Check sheet for the modelled part. Datum: model origin and axes. Units: mm. A direction names the side the tool comes from. Give positions to 0.01 mm unless a question says otherwise; leave off trailing zeros. Write each loop counter-clockwise with the first axis right and the second up, starting at its lowest first coordinate (ties: lowest second). Pieces come first, ordered by that corner, then holes. Notation, with made-up numbers: M 33.5,-31 L 37.5,-31 A14 cw 37.5,-13 Z; hole C -5.75,-12 d8. An arc over 180 degrees is marked long. Write item = value, one per line. Start each with the question number.
1) Mould release check, pull along X, two halves, no side actions. Record for faces 1 (the flat face through (4.4, 8.255, -0.1)), 2 (the flat face through (1.905, 4, -5)), 3 (the cylindrical face through (-0.07, 0.63, -11.43)): released by +X, released by -X, zero draft, split by the parting line, or undercut.
2) Access from +Z, -Z, +X, -X, +Y, -Y to the whole of each face (thin tool, end or side, straight path). Record for faces 4 (the cylindrical face through (-6.35, 3.93, 0.11)), 5 (the cylindrical face through (6.35, 3.93, -0.11)), 6 (the flat face through (1.905, 4, 5)).
3) Cross-section at A-A, the plane x = 0. Record the cut outline in (y, z), plus the area to 3 significant figures.
4) Scan lines: line 1 along Z through (x, y) = (0, 0.8); line 2 along Y through (x, z) = (-1, 3.5); line 3 along Z through (x, y) = (-3.5, 4). Record each from-to range of solid material in increasing order. Write a range as [from, to].
5) Go/stop test with flat-tipped pins: pin 1 (1.1 mm diameter, centred on y = 5.5, z = -5.5, fed in from -X); pin 2 (1.5 mm diameter, centred on x = 0, z = -6.731, fed in from +Y); pin 3 (0.7 mm diameter, centred on y = 2.5, z = -5.5, fed in from +X); pin 4 (1.6 mm diameter, centred on y = 4, z = 5.5, fed in from -X). Record where each tip stops, or that it passes through.
Autodesk Inventor part; units mm, degrees
ref_plane "Work Plane1" through (0, 8.255, 0) normal (0, 1, 0) x (1, 0, 0)
ref_plane "YZ Plane" through (0, 0, 0) normal (1, 0, 0) x (0, 1, 0)
ref_plane "XZ Plane" through (0, 0, 0) normal (0, 1, 0) x (-1, 0, 0)
sketch "Sketch1" plane through (0, 0, 0) normal (0, 1, 0) x (-1, 0, 0)
  arc A0 (-4.4691, 4.5111) -> (4.4691, 4.5111) centre (0, 0) ccw
  arc A1 (3.1656, 8.0108) -> (-3.1656, 8.0108) centre (0, 8.255) ccw
  circle A2 centre (0, -8.255) radius 3.175
  line L0 (0, 0) -> (3.175, 0)
  arc A3 (3.1656, 8.0108) -> (4.4691, 4.5111) centre (7.5974, 7.6688) ccw
  arc A4 (-4.4691, 4.5111) -> (-3.1656, 8.0108) centre (-7.5974, 7.6688) ccw
  arc A5 (-3.1656, -8.0108) -> (-4.4691, -4.5111) centre (-7.5974, -7.6688) ccw
  arc A6 (4.4691, -4.5111) -> (3.1656, -8.0108) centre (7.5974, -7.6688) ccw
  dimension "d0" = 12.7
  dimension "d2" = 6.35
  dimension "d4" = 6.35
  dimension "d5" = 8.89
  dimension "d6" = 16.51
extrude "Extrusion1" add sketch "Sketch1" along normal blind 1.27
sketch "Sketch2" plane through (0, 1.27, 0) normal (0, 1, 0) x (1, 0, 0)
  line L0 (1.905, -7.3814) -> (-1.905, -7.3814)
  line L1 (-1.905, -7.3814) -> (-1.905, 7.3814)
  line L2 (-1.905, 7.3814) -> (1.905, 7.3814)
  line L3 (1.905, 7.3814) -> (1.905, -7.3814)
  line L4 (1.905, -7.3814) -> (-1.905, 7.3814) construction
  line L5 (-1.905, -7.3814) -> (1.905, 7.3814) construction
  arc A0 (1.905, -4.6407) -> (1.905, 4.6407) centre (0, 0) ccw
  arc A1 (-1.905, 4.6407) -> (-1.905, -4.6407) centre (0, 0) ccw
  arc A2 (1.905, -6.0575) -> (1.905, 6.0575) centre (0, 0) ccw
  arc A3 (-1.905, 6.0575) -> (-1.905, -6.0575) centre (0, 0) ccw
  dimension "d11" = 3.81
  dimension "d34" = 5.0165
  dimension "d35" = 6.35
  dimension "d36" = 5.0165
  dimension "d37" = 6.35
extrude "Extrusion2" add sketch "Sketch2" along normal blind 5.3975 contours L3 A0 A2 | A3 L1 A1
sketch "Sketch3" plane through (0, 6.6675, 0) normal (0, 1, 0) x (1, 0, 0)
  arc A0 (-1.905, 4.6407) -> (-1.905, -4.6407) centre (0, 0) ccw
  line L0 (-1.905, 4.6407) -> (-1.905, 6.0575)
  arc A1 (-1.905, 6.0575) -> (-1.905, -6.0575) centre (0, 0) ccw
  line L1 (-1.905, -6.0575) -> (-1.905, -4.6407)
  line L2 (1.905, -4.6407) -> (1.905, -6.0575)
  arc A2 (1.905, -6.0575) -> (1.905, 6.0575) centre (0, 0) ccw
  line L3 (1.905, 6.0575) -> (1.905, 4.6407)
  arc A3 (1.905, -4.6407) -> (1.905, 4.6407) centre (0, 0) ccw
ref_plane "Work Plane1" through (0, 8.255, 0) normal (0, 1, 0) x (1, 0, 0)
sketch "Sketch4" plane through (0, 8.255, 0) normal (0, 1, 0) x (1, 0, 0)
  arc A0 (0.508, -4.9907) -> (0.508, 4.9907) centre (0, 0) ccw
  arc A1 (0.508, -4.0961) -> (0.508, 4.0961) centre (0, 0) ccw
  line L0 (0.508, -4.9907) -> (0.508, -4.0961)
  line L1 (0.508, 4.0961) -> (0.508, 4.9907)
sketch "Sketch5" plane through (0, 8.255, 0) normal (0, 1, 0) x (1, 0, 0)
  line L0 (-0.508, -4.0961) -> (-0.508, -4.9907)
  arc A0 (-0.508, 4.0961) -> (-0.508, -4.0961) centre (0, 0) ccw
  arc A1 (-0.508, 4.9907) -> (-0.508, -4.9907) centre (0, 0) ccw
  line L1 (-0.508, 4.0961) -> (-0.508, 4.9907)
loft "Loft1" add profiles "Sketch4" section 1 edges at (1.905, 6.6675, 5.3491) (6.35, 6.6675, 0) (1.905, 6.6675, -5.3491) (5.0165, 6.6675, 0)
loft "Loft2" add profiles "Sketch5" section 1 edges at (-5.0165, 6.6675, 0) (-1.905, 6.6675, -5.3491) (-6.35, 6.6675, 0) (-1.905, 6.6675, 5.3491)
sketch "Sketch6" plane through (0, 1.27, 0) normal (0, 1, 0) x (1, 0, 0)
  line L0 (0, 0) -> (-3.0006, 0)
  point P0 (0, -6.731)
  point P1 (0, 6.731)
  dimension "d26" = 13.462
hole "Hole1" at (0, 1.27, 6.731) at (0, 1.27, -6.731) direction (0, -1, 0) diameter 2.4384 end through all
properties part number "CasterEnclosure" material "ABS Plastic"
Reply:
q1.face_1 = zero draft
q1.face_2 = undercut
q1.face_3 = split by the parting line
q2.face_4 = -X, +Y
q2.face_5 = +X, +Y
q2.face_6 = +Z, -Z
q3.outline = M 0,-11.43 L 1.27,-11.43 L 1.27,-7.95 L 0,-7.95 Z; M 0,-5.51 L 1.27,-5.51 L 1.27,5.51 L 0,5.51 Z; M 0,7.95 L 1.27,7.95 L 1.27,11.43 L 0,11.43 Z
q3.area = 22.8 mm2
q4.line_1 = [-11.43, -7.95], [-5.51, 5.51], [7.95, 11.43]
q4.line_2 = [0, 1.27]
q4.line_3 = [-5.3, -3.59], [3.59, 5.3]
q5.pin_1 = -3.98
q5.pin_2 = through
q5.pin_3 = 3.71
q5.pin_4 = -4.27
